from build123d import *

# Parameters (mm, degrees)
SKETCH2_W           = 175
SKETCH2_H           = 65
BOSS_EXTRUDE1_DEPTH = 35
SKETCH3_W           = 170
SKETCH3_H           = 60
CUT_EXTRUDE1_DEPTH  = 32.5
SKETCH4_W           = 15
SKETCH4_H           = 8
CUT_EXTRUDE3_DEPTH  = 172.5
SKETCH5_W           = 63
SKETCH5_H           = 2
CUT_EXTRUDE5_DEPTH  = 173.5
SKETCH7_W           = 60
SKETCH7_H           = 2
CUT_EXTRUDE6_DEPTH  = 2.5


with BuildPart() as part:
    # Sketch2 → Boss-Extrude1 (new body)
    with BuildSketch(Plane(origin=(0, 0, 0), x_dir=(1, 0, 0), z_dir=(0, 1, 0))):
        with Locations((-4.104793892, 27.168582034)):
            Rectangle(SKETCH2_W, SKETCH2_H)
    extrude(amount=BOSS_EXTRUDE1_DEPTH)

    # Sketch3 → Cut-Extrude1 (cut)
    with BuildSketch(Plane(origin=(0, 35, 0), x_dir=(1, 0, 0), z_dir=(0, 1, 0))):
        with Locations((-4.104793892, 27.168582034)):
            Rectangle(SKETCH3_W, SKETCH3_H)
    extrude(amount=-CUT_EXTRUDE1_DEPTH, mode=Mode.SUBTRACT)

    # Sketch4 → Cut-Extrude3 (cut)
    with BuildSketch(Plane(origin=(83.395206108, 0, 0), x_dir=(0, 0, -1), z_dir=(1, 0, 0))):
        with Locations((12.668582034, 21.5)):
            Rectangle(SKETCH4_W, SKETCH4_H)
    extrude(amount=-CUT_EXTRUDE3_DEPTH, mode=Mode.SUBTRACT)

    # Sketch5 → Cut-Extrude5 (cut)
    with BuildSketch(Plane.ZY.offset(91.604793892)):
        with Locations((-27.168582034, 32)):
            Rectangle(SKETCH5_W, SKETCH5_H)
    extrude(amount=-CUT_EXTRUDE5_DEPTH, mode=Mode.SUBTRACT)

    # Sketch7 → Cut-Extrude6 (cut)
    with BuildSketch(Plane.ZY.offset(91.604793892)):
        with Locations((-27.168582034, 34)):
            Rectangle(SKETCH7_W, SKETCH7_H)
    extrude(amount=-CUT_EXTRUDE6_DEPTH, mode=Mode.SUBTRACT)


solid = part.part
Design review of the part built by this model. Coordinates are the model's own, in mm. A direction names the side the tool comes from. Give positions to 0.01 mm unless a question says otherwise; leave off trailing zeros. Order: outer loops, then holes, each group sorted by start corner. A loop starts at its lowest first (then second) coordinate and runs counter-clockwise, first axis right, second up. Notation, with made-up numbers: (48.5, -29) - (58.5, -29) arc R9 ccw to (58.5, -15) - close; hole circle Ø4 at (19, -15.5). An arc over 180 degrees is marked (long way). Use CSV: the item, a comma, the result in double quotes. Start each with the question number.
Q1. For line 1 (Z direction, x = -17, y = 30.5); line 2 (X direction, y = 29, z = -50.5); line 3 (Y direction, x = -41, z = -3.5), list the stretches that pass through material, from the lowest coordinate up.
Q2. Take a section at A-A (z = -11). State the section outline as (x, y) points.
Q3. Take a section at C-C (y = 12). State the section outline as (x, z) points, and give its area (4 significant figures).
Q4. Take a section at D-D (z = -25.5). State the section outline as (x, y) points.
Q5. For P1, Ø19, axis at x = -6.5, z = -14.5, coming from the +Y side; P2, Ø4, axis at x = -38.5, z = -42.5, coming from the -Y side, all flat-tipped, find the tip position at first contact; note any pin that passes through.
Q6. Draft analysis for pull direction X (two halves, no side actions). For faces 4 (the face through (-5, 0, -28)), 5 (the face through (83.395, 17, -27)), 6 (the face through (80.895, 17, -27)), state which applies: pulls with the +X half, pulls with the -X half, needs draft (parallel to the pull), parting line crosses it, or undercut.
Q7. Machinability: for faces 1 (the face through (-5, 33, 3)), 2 (the face through (-89.105, 17, -27)), 3 (the face through (-91.605, 17, -27)), which of the approach directions +Z, -Z, +X, -X, +Y, -Y give a long, thin tool a straight path to every point of the face, cutting with its end or side? Answer none if there is none.
Q8. Take a section at B-B (x = -78.5). State the section outline as (y, z) points.
Calculated:
1,line 1,"z = -59.67 to -57.17, 2.83 to 5.33"
1,line 2,"x = -91.6 to -89.1, 80.9 to 83.4"
1,line 3,"y = 0 to 2.5"
2,outline,"(-91.6, 0) - (83.4, 0) - (83.4, 17.5) - (80.9, 17.5) - (80.9, 2.5) - (-89.1, 2.5) - (-89.1, 31) - (-91.6, 31) - close; (80.9, 25.5) - (83.4, 25.5) - (83.4, 35) - (80.9, 35) - (80.9, 33) - (81.9, 33) - (81.9, 31) - (80.9, 31) - close"
3,outline,"(-91.6, -59.67) - (83.4, -59.67) - (83.4, 5.33) - (-91.6, 5.33) - close; hole (-89.1, -57.17) - (80.9, -57.17) - (80.9, 2.83) - (-89.1, 2.83) - close"
3,area,"1,175 mm²"
4,outline,"(-91.6, 0) - (83.4, 0) - (83.4, 35) - (80.9, 35) - (80.9, 33) - (81.9, 33) - (81.9, 31) - (80.9, 31) - (80.9, 2.5) - (-89.1, 2.5) - (-89.1, 31) - (-91.6, 31) - close"
5,P1,"stops at y = 2.5"
5,P2,"stops at y = 0"
6,face 4,"needs draft"
6,face 5,"pulls with the +X half"
6,face 6,"undercut"
7,face 1,"-X"
7,face 2,"+Y"
7,face 3,"+Z, -Z, -X, +Y, -Y"
8,outline,"(0, -59.67) - (35, -59.67) - (35, -57.17) - (33, -57.17) - (33, -58.67) - (31, -58.67) - (31, -57.17) - (2.5, -57.17) - (2.5, 2.83) - (31, 2.83) - (31, 4.33) - (33, 4.33) - (33, 2.83) - (35, 2.83) - (35, 5.33) - (0, 5.33) - close"
